Input: part model. Units: mm. Frame: model coordinates. A direction names the side the tool comes from. Coordinates: 2 decimals unless noted, no trailing zeros. Order: outer loops, then holes, each group sorted by start corner. A loop starts at its lowest first (then second) coordinate and runs counter-clockwise, first axis right, second up. Notation, with made-up numbers: (68.5, 58.25) - (106.5, 58.25) arc R15 ccw to (106.5, 71.25) - close; hole circle Ø8 at (84, -30.75). An arc over 180 degrees is marked (long way). One line per question, with ' | ' between items.
from build123d import *

# Parameters (mm, degrees)
F0_W     = 350
F0_H     = 50
F1_DEPTH = 20
F2_W     = 8
F2_H     = 50
F3_DEPTH = 10
F4_W     = 8
F4_H     = 50
F5_DEPTH = 10


with BuildPart() as f1:
    # F0 (on Front) → F1 (new body)
    with BuildSketch(Plane.XZ):
        Rectangle(F0_W, F0_H)
    extrude(amount=F1_DEPTH)

    # F2 (on face) → F3 (join)
    with BuildSketch(Plane(origin=(-175, 0, 0), x_dir=(0, -1, 0), z_dir=(-1, 0, 0))):
        with Locations((10, 0)):
            Rectangle(F2_W, F2_H)
    extrude(amount=F3_DEPTH)

    # F4 (on face) → F5 (join)
    with BuildSketch(Plane.YZ.offset(175)):
        with Locations((-10, 0)):
            Rectangle(F4_W, F4_H)
    extrude(amount=F5_DEPTH)


solid = f1.part
Item 1: Ray query, line 1 (X direction, y = -17, z = 15). Return the intervals inside material, ascending.
Data:
line 1: -175 to 175
Item 2: Section A-A on z = -14. Return the cut outline in (x, y).
Data:
outline: (-185, -14) - (-175, -14) - (-175, -20) - (175, -20) - (175, -14) - (185, -14) - (185, -6) - (175, -6) - (175, 0) - (-175, 0) - (-175, -6) - (-185, -6) - close
Item 3: Contact query for flat-ended pins moving along their axis: P1, Ø1.8, axis at y = -16.5, z = 4, coming from the +X side; P2, Ø8, axis at x = 180.5, z = 12, coming from the +Y side; P3, Ø3, axis at y = -18.5, z = -12.5, coming from the -X side. Output: stop coordinate, or through.
Data:
P1: x = 175 | P2: y = -6 | P3: x = -175
Item 4: Access query for faces 1 (the face through (-175, -3, 0)), 2 (the face through (-180, -14, 0)), 3 (the face through (-2, -20, 0)), 4 (the face through (175, -17, 0)), 5 (the face through (180, -6, 0)). Directions: +Z, -Z, +X, -X, +Y, -Y. A direction counts if a zero-diameter tool reaches every point of the face in a straight line with its end or side. Return the directions, or none.
Data:
face 1: +Z, -Z, -X, +Y | face 2: +Z, -Z, -X, -Y | face 3: +Z, -Z, +X, -X, -Y | face 4: +Z, -Z, +X, -Y | face 5: +Z, -Z, +X, +Y
